For this review, take the finished solid that the model builds, in its own axes (mm). Face numbers are marked on the shaded views. A direction names the side the tool comes from. Give positions to 0.01 mm unless a question says otherwise; leave off trailing zeros. Order: outer loops, then holes, each group sorted by start corner. A loop starts at its lowest first (then second) coordinate and runs counter-clockwise, first axis right, second up. Notation, with made-up numbers: (38.25, 47.25) - (70.25, 47.25) arc R26 cw to (70.25, 80.25) - close; hole circle Ø7 at (34, -30.5). An arc over 180 degrees is marked (long way). Use a Markdown table: item, result. Add a question column.
1) Clearance check with flat-ended pins moving along their axes: P1, Ø1, axis at x = 6, y = 1.5, coming from the +Z side; P2, Ø1.7, axis at x = 1, z = -7.5, coming from the -Y side; P3, Ø1, axis at y = 1, z = -0.5, coming from the -X side. State where each tip first meets the part, or that it passes through.
2) Machinability: for the marked faces 4 and 5, which of the approach directions +Z, -Z, +X, -X, +Y, -Y give a long, thin tool a straight path to every point of the face, cutting with its end or side? Answer none if there is none.
3) Wall thickness on L1, parallel to Z at x = 8, y = 1.7; L2, parallel to Z at x = -7, y = 1.6; L3, parallel to Z at x = 1.5, y = 1.95: over which ranges is each line inside the solid? List them lowest first.
4) We need section B-B on x = -6. Write out the cut boundary in (y, z), then the cut area to 3 significant figures.
5) We need section C-C on y = 1.15. Give the number of separate pieces and of enclosed holes in the cut face, then the cut area to 3 significant figures.
6) We need section D-D on x = 6. Write out the cut boundary in (y, z).
7) Mouldability with a two-part tool opening along X and no side actions: class the marked faces 1, 2 and 3 as released by +X, released by -X, zero draft, split by the parting line, or undercut.
```python
from build123d import *

# Parameters (mm, degrees)
SKETCH1_R                = 18
BOSS_EXTRUDE1_DEPTH      = 2.5
CUT_EXTRUDE4_OUTLINE_W   = 10.16
CUT_EXTRUDE4_OUTLINE_H   = 5.715
CUT_EXTRUDE4_OUTLINE_W_2 = 2.312550402
CUT_EXTRUDE4_OUTLINE_H_2 = 3.94124845
CUT_EXTRUDE4_OUTLINE_W_3 = 2.75
CUT_EXTRUDE4_OUTLINE_H_3 = 3.7
CUT_EXTRUDE4_OUTLINE_W_4 = 9.525
CUT_EXTRUDE4_OUTLINE_H_4 = 5.6
CUT_EXTRUDE4_DEPTH       = 2


# Read off the part's stored shape, not the designer's step: Cut-Extrude4
with BuildPart() as part:
    # Sketch1 → Boss-Extrude1 (new body)
    with BuildSketch(Plane(origin=(0, 0, 0), x_dir=(1, 0, 0), z_dir=(0, 1, 0))):
        with Locations(Location((0, 0, 0), (0, 0, 270))):
            Circle(SKETCH1_R)
    extrude(amount=BOSS_EXTRUDE1_DEPTH)

    # Cut-Extrude4 outline → Cut-Extrude4 (cut)
    with BuildSketch(Plane(origin=(0, 0, 0), x_dir=(1, 0, 0), z_dir=(0, 1, 0))):
        with Locations((0, -6.35)):
            Rectangle(CUT_EXTRUDE4_OUTLINE_W, CUT_EXTRUDE4_OUTLINE_H)
        with Locations((6.578724799, 4.629375775)):
            Rectangle(CUT_EXTRUDE4_OUTLINE_W_2, CUT_EXTRUDE4_OUTLINE_H_2)
        with Locations((6.36, 0)):
            Rectangle(CUT_EXTRUDE4_OUTLINE_W_3, CUT_EXTRUDE4_OUTLINE_H_3)
        Polygon((-4.297709584, -13.968636918), (-2.881780884, -10.550282647), (-5.422449598, -9.497903208), (-6.838378298, -12.916257479), align=None)
        Polygon((2.881780884, 10.550282647), (5.422449598, 9.497903208), (6.838378298, 12.916257479), (4.297709584, 13.968636918), align=None)
        Polygon((-0.535919412, -14.604996247), (-0.052972501, -10.93665026), (-2.77944587, -10.577703232), (-3.262392781, -14.246049219), align=None)
        Polygon((0.052972501, 10.93665026), (2.77944587, 10.577703232), (3.262392781, 14.246049219), (0.535919412, 14.604996247), align=None)
        Polygon((-10.706244136, -9.948339635), (-7.770836777, -7.695922348), (-9.444930707, -5.514200662), (-12.380338066, -7.766617949), align=None)
        Polygon((-7.766617949, -12.380338066), (-5.514200662, -9.444930707), (-7.695922348, -7.770836777), (-9.948339635, -10.706244136), align=None)
        with Locations((-3.175, 0)):
            Rectangle(CUT_EXTRUDE4_OUTLINE_W_3, CUT_EXTRUDE4_OUTLINE_H_3)
        with Locations((-6.35, 0)):
            Rectangle(CUT_EXTRUDE4_OUTLINE_W_3, CUT_EXTRUDE4_OUTLINE_H_3)
        with Locations((-9.525, 0)):
            Rectangle(CUT_EXTRUDE4_OUTLINE_W_3, CUT_EXTRUDE4_OUTLINE_H_3)
        Rectangle(CUT_EXTRUDE4_OUTLINE_W_3, CUT_EXTRUDE4_OUTLINE_H_3)
        with Locations((3.18, 0)):
            Rectangle(CUT_EXTRUDE4_OUTLINE_W_3, CUT_EXTRUDE4_OUTLINE_H_3)
        with Locations((9.54, 0)):
            Rectangle(CUT_EXTRUDE4_OUTLINE_W_3, CUT_EXTRUDE4_OUTLINE_H_3)
        with Locations((0, 6.6)):
            Rectangle(CUT_EXTRUDE4_OUTLINE_W_4, CUT_EXTRUDE4_OUTLINE_H_4)
        Polygon((-6.838378298, 12.916257479), (-5.422449598, 9.497903208), (-2.881780884, 10.550282647), (-4.297709584, 13.968636918), align=None)
        Polygon((5.422449598, -9.497903208), (2.881780884, -10.550282647), (4.297709584, -13.968636918), (6.838378298, -12.916257479), align=None)
        Polygon((-3.262392781, 14.246049219), (-2.77944587, 10.577703232), (-0.052972501, 10.93665026), (-0.535919412, 14.604996247), align=None)
        Polygon((2.77944587, -10.577703232), (0.052972501, -10.93665026), (0.535919412, -14.604996247), (3.262392781, -14.246049219), align=None)
        Polygon((12.380338066, -7.766617949), (9.444930707, -5.514200662), (7.770836777, -7.695922348), (10.706244136, -9.948339635), align=None)
        Polygon((9.948339635, -10.706244136), (7.695922348, -7.770836777), (5.514200662, -9.444930707), (7.766617949, -12.380338066), align=None)
    extrude(amount=CUT_EXTRUDE4_DEPTH, mode=Mode.SUBTRACT)


solid = part.part
```
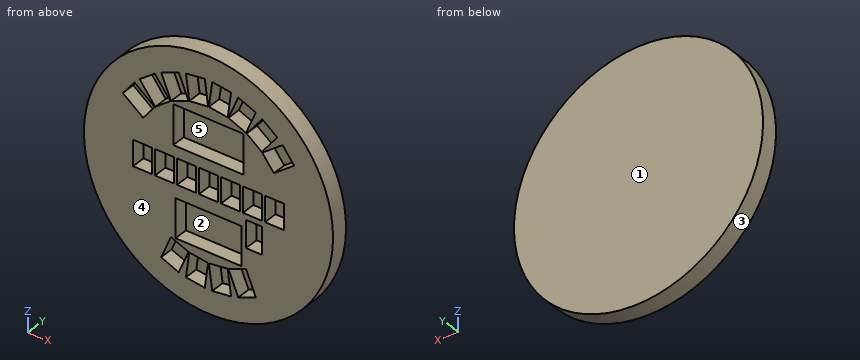
Checked values:
| question | item | result |
|---|---|---|
| 1 | P1 | z = 17.14 |
| 1 | P2 | y = 2 |
| 1 | P3 | x = -18 |
| 2 | face 4 | +Z, -Z, +X, -X, -Y |
| 2 | face 5 | -Y |
| 3 | L1 | -16.12 to 7.4, 7.87 to 8.17, 12.2 to 16.12 |
| 3 | L2 | -16.58 to -1.85, 1.85 to 8.3, 11.38 to 16.58 |
| 3 | L3 | -17.94 to -14.48, -10.75 to -9.4, -3.8 to 3.49, 9.21 to 10.75, 14.48 to 17.94 |
| 4 | outline | (0, -16.97) - (2.5, -16.97) - (2.5, 16.97) - (0, 16.97) - (0, 13.26) - (2, 13.26) - (2, 10.89) - (0, 10.89) - (0, 10.08) - (2, 10.08) - (2, 9.07) - (0, 9.07) - (0, 1.85) - (2, 1.85) - (2, -1.85) - (0, -1.85) - (0, -10.89) - (2, -10.89) - (2, -13.26) - (0, -13.26) - close |
| 4 | area | 66.0 mm² |
| 5 | separate pieces | 1 |
| 5 | enclosed holes | 22 |
| 5 | area | 704 mm² |
| 6 | outline | (0, -16.97) - (2.5, -16.97) - (2.5, 16.97) - (0, 16.97) - (0, 13.26) - (2, 13.26) - (2, 10.89) - (0, 10.89) - (0, 10.08) - (2, 10.08) - (2, 9.07) - (0, 9.07) - (0, 1.85) - (2, 1.85) - (2, -1.85) - (0, -1.85) - (0, -2.66) - (2, -2.66) - (2, -6.6) - (0, -6.6) - (0, -10.89) - (2, -10.89) - (2, -13.26) - (0, -13.26) - close |
| 7 | face 1 | zero draft |
| 7 | face 2 | undercut |
| 7 | face 3 | split by the parting line |
